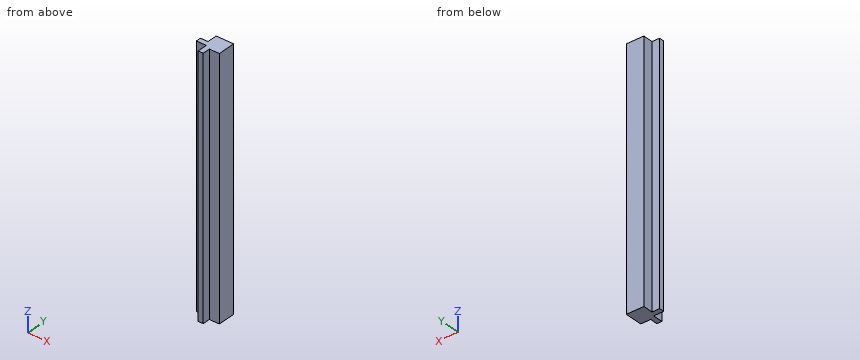
Autodesk Inventor part; units mm, degrees
ref_plane "Arbeitsebene1" through (0, 0, 100) normal (0, 0, 1) x (1, 0, 0)
ref_plane "YZ Plane" through (0, 0, 0) normal (1, 0, 0) x (0, 1, 0)
ref_plane "XZ Plane" through (0, 0, 0) normal (0, 1, 0) x (-1, 0, 0)
sketch "Skizze1" plane through (0, 0, 0) normal (0, 0, 1) x (1, 0, 0)
  line L0 (0, 0) -> (10, 0)
  line L1 (10, 0) -> (10, 10)
  line L2 (10, 10) -> (0, 10)
  line L3 (0, 10) -> (0, 0)
extrude "Extrusion1" add sketch "Skizze1" along normal blind 100
sketch "Skizze2" plane through (0, 0, 0) normal (0, 0, 1) x (1, 0, 0)
  line L0 (0, 0) -> (4, 0)
  line L1 (4, 0) -> (4, 4)
  line L2 (4, 4) -> (0, 4)
  line L3 (0, 4) -> (0, 0)
extrude "Extrusion2" cut sketch "Skizze2" along normal blind 100
sketch "Skizze3" plane through (0, 0, 0) normal (0, 0, 1) x (1, 0, 0)
  line L0 (-3, 6) -> (3, 6)
  line L1 (3, 6) -> (3, 10)
  line L2 (3, 10) -> (-3, 10)
  line L3 (-3, 10) -> (-3, 6)
extrude "Extrusion3" cut sketch "Skizze3" along normal blind 100
sketch "Skizze4" plane through (0, 0, 0) normal (0, 0, 1) x (1, 0, 0)
  line L0 (-3, -10) -> (3, -10)
  line L1 (3, -10) -> (3, -6)
  line L2 (3, -6) -> (-3, -6)
  line L3 (-3, -6) -> (-3, -10)
extrude "Extrusion4" cut sketch "Skizze4" along normal blind 100
sketch "Skizze5" plane through (0, 0, 0) normal (0, 0, 1) x (1, 0, 0)
  line L0 (-10, -3) -> (-6, -3)
  line L1 (-6, -3) -> (-6, 3)
  line L2 (-6, 3) -> (-10, 3)
  line L3 (-10, 3) -> (-10, -3)
extrude "Extrusion5" cut sketch "Skizze5" along normal blind 100
sketch "Skizze6" plane through (0, 0, 0) normal (0, 0, 1) x (1, 0, 0)
  line L0 (6, -3) -> (10, -3)
  line L1 (10, -3) -> (10, 3)
  line L2 (10, 3) -> (6, 3)
  line L3 (6, 3) -> (6, -3)
extrude "Extrusion6" cut sketch "Skizze6" along normal blind 100
ref_plane "Arbeitsebene1" through (0, 0, 100) normal (0, 0, 1) x (1, 0, 0)
sketch "Skizze7" plane through (0, 0, 0) normal (0, 0, 1) x (1, 0, 0)
  circle A0 centre (0, 0) radius 2.5
extrude "Extrusion7" cut sketch "Skizze7" along normal blind 10
sketch "Skizze8" plane through (0, 0, 100) normal (0, 0, 1) x (1, 0, 0)
  circle A0 centre (0, 0) radius 2.5
extrude "Extrusion8" cut sketch "Skizze8" along normal blind 10
properties part number "Aluprofil_20x20_H100"
The listing builds one solid part. Answer for the finished solid, in the listing's coordinates (mm). Give positions to 0.01 mm unless a question says otherwise; leave off trailing zeros. Write each loop counter-clockwise with the first axis right and the second up, starting at its lowest first coordinate (ties: lowest second). Pieces come first, ordered by that corner, then holes. Notation, with made-up numbers: (-19.75, 25) -> (38.25, 25) arc R21 cw to (38.25, 59) -> close; hole circle Ø2 at (51, 7.5). An arc over 180 degrees is marked (long way). Use one line per item in the form item = value.
1) Each of these flat-tipped pins is pushed along its axis until it touches: P1, Ø1.2, axis at x = 1.5, z = 48.5, coming from the -Y side; P2, Ø1, axis at x = 8.5, z = 30.5, coming from the -Y side; P3, Ø1.2, axis at y = 8, z = 57, coming from the -X side. Where does it stop, or does it pass through?
Result:
P1 = 4
P2 = 3
P3 = 3
2) Section B-B on x = 1.25 is taken. Write down the section's boundary in (y, z), plus the area to 3 significant figures.
Result:
outline = (4, 0) -> (6, 0) -> (6, 100) -> (4, 100) -> close
area = 200 mm²
3) Straight lines are drawn through the part: probe 1 along X at (y, z) = (9, 65); probe 2 along X at (y, z) = (1, 88.5). For each, find the intervals that lie inside material, in ascending order.
Result:
probe_1 = 3 to 10
probe_2 = 4 to 6
4) Section A-A on z = 12 is taken. Write down the section's boundary in (x, y).
Result:
outline = (0, 4) -> (4, 4) -> (4, 0) -> (6, 0) -> (6, 3) -> (10, 3) -> (10, 10) -> (3, 10) -> (3, 6) -> (0, 6) -> close
5) Section C-C on y = 8 is taken. Write down the section's boundary in (x, z), plus the area to 3 significant figures.
Result:
outline = (3, 0) -> (10, 0) -> (10, 100) -> (3, 100) -> close
area = 700 mm²
